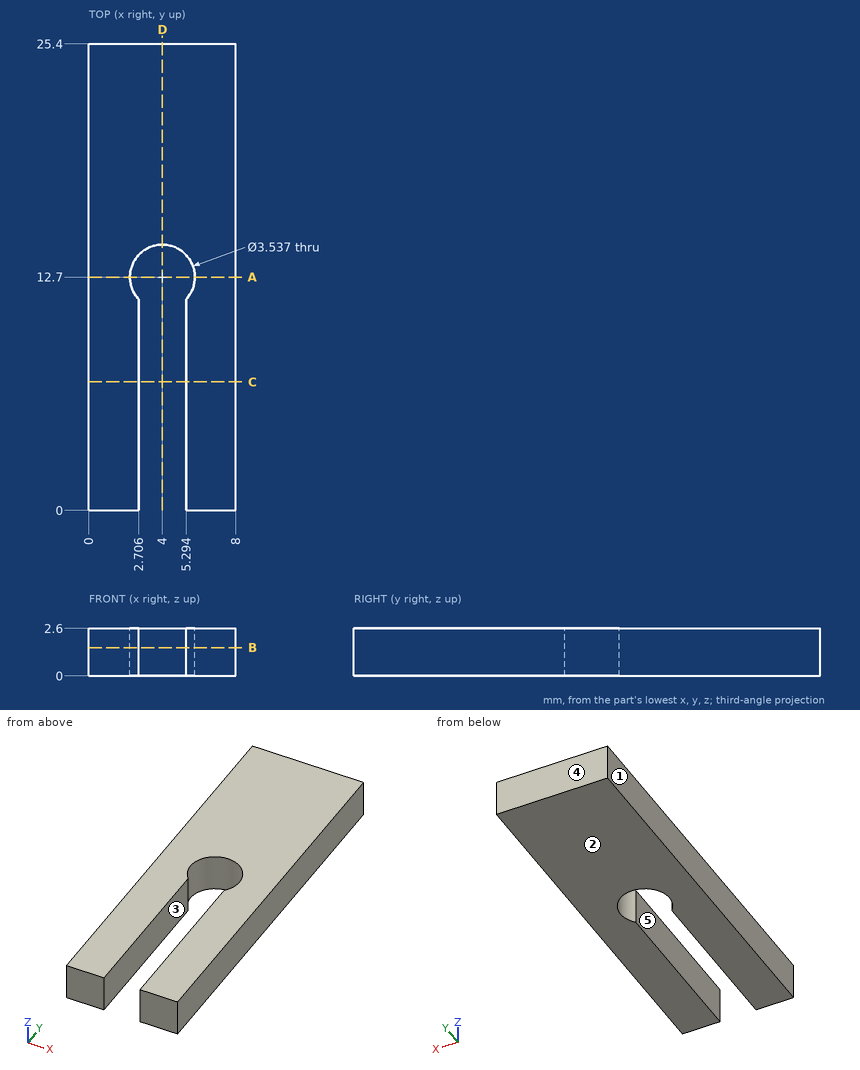
Here's the drawing with two shaded views (mm, measured from the low corner). I have some questions. A direction names the side the tool comes from. Round coordinates to 2 decimals unless told otherwise and drop trailing zeros. Loops run counter-clockwise (first coordinate to the right, second up) from the corner with the lowest first, then second, coordinate; pieces in that order, holes last. Notation, with made-up numbers: (55.5, 15.5) - (66.5, 15.5) arc R13 ccw to (66.5, 39.5) - close; hole circle Ø10 at (58, 16). An arc over 180 degrees is marked (long way). Write item = value, one per line.
1) Imagine slicing it at A-A (y = 12.7). Please give me the cut outline in (x, z), and give its area (3 significant figures).
Computed:
outline = (0, 0) - (2.23, 0) - (2.23, 2.6) - (0, 2.6) - close; (5.77, 0) - (8, 0) - (8, 2.6) - (5.77, 2.6) - close
area = 11.6 mm2
2) If we mould it in two halves opening along X, with no side actions, what happens to the marked faces 1, 2 and 3? For each: pulls with the +X half, pulls with the -X half, needs draft (parallel to the pull), parting line crosses it, or undercut.
Computed:
face_1 = pulls with the -X half
face_2 = needs draft
face_3 = undercut
3) On a 3-axis mill with a long thin cutter (end or side, diameter ignored), from which of +Z, -Z, +X, -X, +Y, -Y can I reach the whole of each face in a straight line? I mean the marked faces 4 and 5. Say none if no direction works.
Computed:
face_4 = +Z, -Z, +X, -X, +Y
face_5 = +Z, -Z, -Y
4) Imagine slicing it at B-B (z = 1.55). Please give me the cut outline in (x, y).
Computed:
outline = (0, 0) - (2.71, 0) - (2.71, 11.49) arc R1.77 cw (long way) to (5.29, 11.49) - (5.29, 0) - (8, 0) - (8, 25.4) - (0, 25.4) - close
5) Imagine slicing it at D-D (x = 4). Please give me the cut outline in (y, z), and give its area (3 significant figures).
Computed:
outline = (14.47, 0) - (25.4, 0) - (25.4, 2.6) - (14.47, 2.6) - close
area = 28.4 mm2
6) I need wall thicknesses on line 1 along X through (y, z) = (3.25, 1.2); line 2 along X through (y, z) = (12.7, 0.7); line 3 along Y through (x, z) = (4, 0.8). Which ranges of each line are inside material? Lowest first, please. Write a range as from..to.
Computed:
line_1 = 0..2.71, 5.29..8
line_2 = 0..2.23, 5.77..8
line_3 = 14.47..25.4
7) Imagine slicing it at C-C (y = 7). Please give me the cut outline in (x, z).
Computed:
outline = (0, 0) - (2.71, 0) - (2.71, 2.6) - (0, 2.6) - close; (5.29, 0) - (8, 0) - (8, 2.6) - (5.29, 2.6) - close
